Work out the finished part from the listing and answer in its coordinate system (mm). A direction names the side the tool comes from. Round coordinates to 2 decimals unless told otherwise and drop trailing zeros. Loops run counter-clockwise (first coordinate to the right, second up) from the corner with the lowest first, then second, coordinate; pieces in that order, holes last. Notation, with made-up numbers: M 5,43 L 36,43 A20 ccw 36,49 Z; hole C 36,55 d10. An arc over 180 degrees is marked long. One line per item, written item: value.
```python
from build123d import *

# Parameters (mm, degrees)
SKETCH1_R           = 1
BOSS_EXTRUDE1_DEPTH = 28
SKETCH2_W           = 5.706880649
SKETCH2_H           = 7
CUT_EXTRUDE1_DEPTH  = 5
SKETCH3_R           = 2
CUT_EXTRUDE2_DEPTH  = 5


with BuildPart() as part:
    # Sketch1 → Boss-Extrude1 (new body)
    with BuildSketch(Plane(origin=(0, 0, 0), x_dir=(1, 0, 0), z_dir=(0, 1, 0))):
        with BuildLine():
            ThreePointArc((0.266683504, 3), (-3.465367303, 4), (-0.733316496, 1.267949192))
            Line((-0.733316496, 1.267949192), (-0.733316496, -9))
            Line((-0.733316496, -9), (0.266683504, -9))
            Line((0.266683504, -9), (0.266683504, 3))
        make_face()
        with Locations((-1.733316496, 3)):
            Circle(SKETCH1_R, mode=Mode.SUBTRACT)
    extrude(amount=BOSS_EXTRUDE1_DEPTH)

    # Sketch2 → Cut-Extrude1 (cut, through all)
    with BuildSketch(Plane(origin=(0.266683504, 0, 0), x_dir=(0, 0, -1), z_dir=(1, 0, 0))):
        with Locations((3.853440325, 24.5)):
            Rectangle(SKETCH2_W, SKETCH2_H)
        with Locations((3.853440325, 10.5)):
            Rectangle(SKETCH2_W, SKETCH2_H)
    extrude(amount=-CUT_EXTRUDE1_DEPTH, mode=Mode.SUBTRACT)

    # Sketch3 → Cut-Extrude2 (cut, through all)
    with BuildSketch(Plane(origin=(0.266683504, 0, 0), x_dir=(0, 0, -1), z_dir=(1, 0, 0))):
        with Locations((-5, 23)):
            Circle(SKETCH3_R)
        with Locations((-5, 5)):
            Circle(SKETCH3_R)
    extrude(amount=-CUT_EXTRUDE2_DEPTH, mode=Mode.SUBTRACT)


solid = part.part
```
1) Find section D-D (x = -2.4). Give the vertices of the cut face in (y, z), then the cut area to 3 significant figures.
Check values:
outline: M 0,-4.89 L 7,-4.89 L 7,-3.75 L 0,-3.75 Z; M 0,-2.25 L 7,-2.25 L 7,-1.11 L 0,-1.11 Z; M 14,-4.89 L 21,-4.89 L 21,-3.75 L 14,-3.75 Z; M 14,-2.25 L 21,-2.25 L 21,-1.11 L 14,-1.11 Z
area: 31.9 mm2
2) Find section B-B (z = 5). Give the vertices of the cut face in (x, y), then the cut area to 3 significant figures.
Check values:
outline: M -0.73,0 L 0.27,0 L 0.27,3 L -0.73,3 Z; M -0.73,7 L 0.27,7 L 0.27,21 L -0.73,21 Z; M -0.73,25 L 0.27,25 L 0.27,28 L -0.73,28 Z
area: 20.0 mm2
3) Find section C-C (y = 5). Give the vertices of the cut face in (x, z).
Check values:
outline: M -0.73,-1.27 A2 ccw long 0.27,-3 L 0.27,3 L -0.73,3 Z; M -0.73,7 L 0.27,7 L 0.27,9 L -0.73,9 Z; hole C -1.73,-3 d2
4) Each of these flat-tipped pins is pushed along its axis until it touches: pin 1 (1.6 mm diameter, centred on x = -1.73, z = -3, fed in from +Y); pin 2 (1.5 mm diameter, centred on x = -3, y = 13.5, fed in from +Z); pin 3 (1.2 mm diameter, centred on x = -2, z = -3.5, fed in from +Y); pin 4 (5 mm diameter, centred on y = 15, z = 3.5, fed in from -X). Where does it stop, or does it pass through?
Check values:
pin 1: through
pin 2: z = -1.13
pin 3: y = 21
pin 4: x = -0.73
5) Find the intervals of material crossed by probe 1 along Y at (x, z) = (-0.2, 5); probe 2 along Z at (x, y) = (-1.65, 5.25); probe 3 along Y at (x, z) = (-0.65, 4.5), in increasing order. Write a range as from..to.
Check values:
probe 1: 0..3, 7..21, 25..28
probe 2: -5..-4, -2..-1
probe 3: 0..3.06, 6.94..21.06, 24.94..28
6) For faces 1 (the face through (-1, 7, -2)), 2 (the face through (-2.47, 17.451, -3.676)), 3 (the face through (0, 24, -1)), determine the directions among +Z, -Z, +X, -X, +Y, -Y from which every point of the face is accessible in a straight line to the end or side of a thin tool.
Check values:
face 1: -Z, +X, -X
face 2: +Y, -Y
face 3: -Z, +X, -X, +Y
7) The mould has two halves that part along X. Classify faces 4 (the face through (0.267, 14, 3)), 5 (the face through (-2.47, 3.451, -3.676)), 6 (the face through (-1, 14, -2)): +X half, -X half, draft (parallel to the pull), parting line (faces both ways), or undercut.
Check values:
face 4: +X half
face 5: undercut
face 6: draft
8) Find section A-A (y = 23). Give the vertices of the cut face in (x, z), then the cut area to 3 significant figures.
Check values:
outline: M -0.73,-1 L 0.27,-1 L 0.27,3 L -0.73,3 Z; M -0.73,7 L 0.27,7 L 0.27,9 L -0.73,9 Z
area: 6.00 mm2
